CAD build for the part. Positions are in the model's coordinates, mm. Face numbers are marked on the shaded views. A direction names the side the tool comes from. Give positions to 0.01 mm unless a question says otherwise; leave off trailing zeros. Order: outer loops, then holes, each group sorted by start corner. A loop starts at its lowest first (then second) coordinate and runs counter-clockwise, first axis right, second up. Notation, with made-up numbers: (69.25, -30) -> (124.25, -30) arc R31 ccw to (124.25, 6) -> close; hole circle Ø10 at (52.25, 57). An arc over 180 degrees is marked (long way). Use one line per item in the form item = value. Start each with the question number.
1) Cut at B-B, the plane z = 0. Give the cut face in (x, y) (3 decimals), and give its area (3 significant figures).
2) Tool access for the marked faces 4, 5, 6, 7 and 8: list every direction of +Z, -Z, +X, -X, +Y, -Y with a clear straight run to the whole face (end or side of a thin tool).
3) Mould opens along Z. For the marked faces 1, 2 and 3 say: pulls with the +Z half, pulls with the -Z half, needs draft (parallel to the pull), parting line crosses it, or undercut.
4) Probe line 1 (X direction, y = -2.3, z = 0) (3 decimals); line 2 (Y direction, x = -1.15, z = 1.95); line 3 (Z direction, x = -1.3, y = -1.1). List the from-to ranges inside material, lowest first.
5) Cut at A-A, the plane x = 0. Give the cut face in (y, z) (3 decimals), and give its area (3 significant figures).
6) Drop flat-ended pins along their axis: P1, Ø1.3, axis at x = 1, y = -1, coming from the -Z side; P2, Ø0.6, axis at x = -1, y = -0.5, coming from the +Z side; P3, Ø1.5, axis at y = -2, z = 0, coming from the -X side. Give the stop position or say it passes through.
7) Cut at C-C, the plane y = -2.35. Give the cut face in (x, z) (3 decimals), and give its area (3 significant figures).
from build123d import *

# Parameters (mm, degrees)
SKETCH1_W           = 5.45
SKETCH1_H           = 5.45
BOSS_EXTRUDE1_DEPTH = 0.7
SKETCH2_W           = 5
SKETCH2_H           = 5
BOSS_EXTRUDE2_DEPTH = 1.2
SKETCH4_R           = 2.45
BOSS_EXTRUDE3_DEPTH = 0.7
SKETCH5_R           = 1.935
SKETCH5_R_2         = 0.35
BOSS_EXTRUDE4_DEPTH = 1.3


with BuildPart() as part:
    # Sketch1 → Boss-Extrude1 (new body)
    with BuildSketch(Plane(origin=(0, 0, 0), x_dir=(1, 0, 0), z_dir=(0, 1, 0))):
        Rectangle(SKETCH1_W, SKETCH1_H)
    extrude(amount=BOSS_EXTRUDE1_DEPTH)

    # Sketch2 → Boss-Extrude2 (add)
    with BuildSketch(Plane.XZ):
        Rectangle(SKETCH2_W, SKETCH2_H)
    extrude(amount=BOSS_EXTRUDE2_DEPTH)

    # Sketch4 → Boss-Extrude3 (add)
    with BuildSketch(Plane.XZ.offset(1.2)):
        with Locations(Location((0, 0, 0), (0, 0, 270))):
            Circle(SKETCH4_R)
    extrude(amount=BOSS_EXTRUDE3_DEPTH)

    # Sketch5 → Boss-Extrude4 (add)
    with BuildSketch(Plane.XZ.offset(1.9)):
        with Locations(Location((0, 0, 0), (0, 0, 270))):
            Circle(SKETCH5_R)
        with Locations(Location((0, 0, 0), (0, 0, 270))):
            Circle(SKETCH5_R_2, mode=Mode.SUBTRACT)
    extrude(amount=BOSS_EXTRUDE4_DEPTH)


solid = part.part
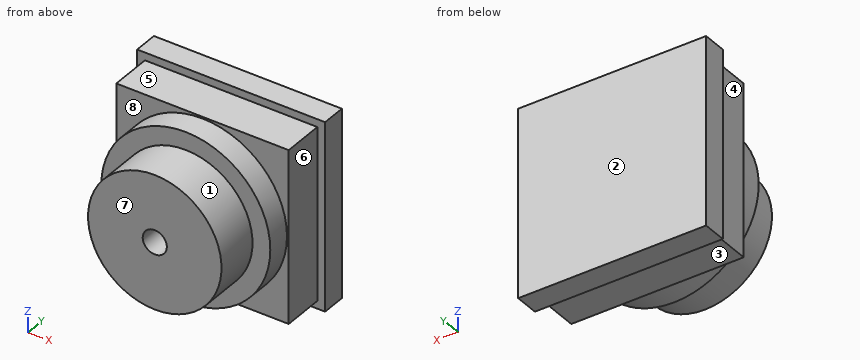
Result:
q1.outline = (-2.725, 0) -> (-2.5, 0) -> (-2.5, -1.2) -> (-2.45, -1.2) -> (-2.45, -1.9) -> (-1.935, -1.9) -> (-1.935, -3.2) -> (-0.35, -3.2) -> (-0.35, -1.9) -> (0.35, -1.9) -> (0.35, -3.2) -> (1.935, -3.2) -> (1.935, -1.9) -> (2.45, -1.9) -> (2.45, -1.2) -> (2.5, -1.2) -> (2.5, 0) -> (2.725, 0) -> (2.725, 0.7) -> (-2.725, 0.7) -> close
q1.area = 17.4 mm²
q2.face_4 = +Z, -Z, -X, -Y
q2.face_5 = +Z, +X, -X, -Y
q2.face_6 = +Z, -Z, +X, -Y
q2.face_7 = +Z, -Z, +X, -X, -Y
q2.face_8 = -Y
q3.face_1 = parting line crosses it
q3.face_2 = needs draft
q3.face_3 = pulls with the -Z half
q4.line_1 = -1.935 to -0.35, 0.35 to 1.935
q4.line_2 = -1.9 to 0.7
q4.line_3 = -2.5 to 2.5
q5.outline = (-3.2, -1.935) -> (-1.9, -1.935) -> (-1.9, -2.45) -> (-1.2, -2.45) -> (-1.2, -2.5) -> (0, -2.5) -> (0, -2.725) -> (0.7, -2.725) -> (0.7, 2.725) -> (0, 2.725) -> (0, 2.5) -> (-1.2, 2.5) -> (-1.2, 2.45) -> (-1.9, 2.45) -> (-1.9, 1.935) -> (-3.2, 1.935) -> (-3.2, 0.35) -> (-1.9, 0.35) -> (-1.9, -0.35) -> (-3.2, -0.35) -> close
q5.area = 17.4 mm²
q6.P1 = -2.5
q6.P2 = 2.5
q6.P3 = -2.45
q7.outline = circle Ø3.87 at (0, 0); hole circle Ø0.7 at (0, 0)
q7.area = 11.4 mm²
